from build123d import *

# Parameters (mm, degrees)
SKETCH1_R            = 28.4
BOSS_EXTRUDE1_DEPTH  = 26
SKETCH2_OUTSIDE_W    = 75.686
SKETCH2_OUTSIDE_H    = 75.686
SKETCH2_OUTSIDE_R    = 15
CUT_EXTRUDE1_DEPTH   = 20
CUT_EXTRUDE2_DEPTH   = 48.844748928
CHAMFER1_SIZE        = 0.5
M5_CLEARANCE_HOLE1_D = 5.5
CIRPATTERN1_COUNT    = 6
SKETCH9_R            = 4
CUT_EXTRUDE3_DEPTH   = 48.844748928


with BuildPart() as part:
    # Sketch1 → Boss-Extrude1 (new body)
    with BuildSketch(Plane.XY):
        with Locations(Location((0, 0, 0), (0, 0, 180))):
            Circle(SKETCH1_R)
    extrude(amount=BOSS_EXTRUDE1_DEPTH)

    # Sketch2 outside → Cut-Extrude1 (cut)
    with BuildSketch(Plane(origin=(0, 0, 0), x_dir=(-1, 0, 0), z_dir=(0, 0, -1))):
        Rectangle(SKETCH2_OUTSIDE_W, SKETCH2_OUTSIDE_H)
        Circle(SKETCH2_OUTSIDE_R, mode=Mode.SUBTRACT)
    extrude(amount=-CUT_EXTRUDE1_DEPTH, mode=Mode.SUBTRACT)

    # Sketch3 → Cut-Extrude2 (cut, through all)
    with BuildSketch(Plane(origin=(0, 0, 0), x_dir=(-1, 0, 0), z_dir=(0, 0, -1))):
        with BuildLine():
            Line((2.5, -6.538348415), (2.5, -9.3))
            Line((2.5, -9.3), (-2.5, -9.3))
            Line((-2.5, -9.3), (-2.5, -6.538348415))
            ThreePointArc((-2.5, -6.538348415), (0, 7), (2.5, -6.538348415))
        make_face()
    extrude(amount=-CUT_EXTRUDE2_DEPTH, mode=Mode.SUBTRACT)

    # Chamfer1
    chamfer1_edges = [part.edges().sort_by_distance(p)[0] for p in [
        (28.4, 0, 26),
        (28.4, 0, 20),
    ]]
    chamfer(chamfer1_edges, length=CHAMFER1_SIZE)

    # M5 Clearance Hole1 (through all)
    with Locations(Plane.XY.offset(26)):
        with Locations((23.75, 0)):
            m5_clearance_hole1 = Hole(M5_CLEARANCE_HOLE1_D / 2)

    # CirPattern1: M5 Clearance Hole1 ×6 about axis
    cirpattern1_axis = Axis((0, 0, 0), (0, 0, 1))
    for i in range(1, CIRPATTERN1_COUNT):
        add(m5_clearance_hole1.rotate(cirpattern1_axis, i * 360 / CIRPATTERN1_COUNT), mode=Mode.SUBTRACT)

    # Sketch9 → Cut-Extrude3 (cut, through all)
    with BuildSketch(Plane(origin=(0, 0, 0), x_dir=(0, 0, -1), z_dir=(1, 0, 0))):
        with Locations((-10.2, 0)):
            Circle(SKETCH9_R)
    extrude(amount=-CUT_EXTRUDE3_DEPTH, mode=Mode.SUBTRACT)


solid = part.part
CAD build for the part. Positions are in the model's coordinates, mm. A direction names the side the tool comes from. Round coordinates to 2 decimals unless told otherwise and drop trailing zeros. Loops run counter-clockwise (first coordinate to the right, second up) from the corner with the lowest first, then second, coordinate; pieces in that order, holes last. Notation, with made-up numbers: (69, 44) - (116, 44) arc R9 ccw to (116, 49) - close; hole circle Ø8 at (-17, 41). An arc over 180 degrees is marked (long way). Put each result on its own line as item: value.
1. Two-plate mould, pull along X, no slides. Class faces 4 (the flat face through (-3.1, 6.5, 0)), 5 (the cylindrical face through (13.144, -18.128, 22.958)), 6 (the cylindrical face through (3.697, -28.158, 22.965)): released by +X, released by -X, zero draft, split by the parting line, or undercut.
Geometry check:
face 4: zero draft
face 5: undercut
face 6: split by the parting line
2. Slice it at A-A on x = 0. List the corners of the cut face in (y, z), and give its area (4 significant figures).
Geometry check:
outline: (-28.4, 20.5) - (-27.9, 20) - (-15, 20) - (-15, 0) - (-9.3, 0) - (-9.3, 26) - (-27.9, 26) - (-28.4, 25.5) - close; (7, 0) - (15, 0) - (15, 20) - (27.9, 20) - (28.4, 20.5) - (28.4, 25.5) - (27.9, 26) - (7, 26) - close
area: 516.5 mm²
3. Slice it at B-B on y = 0. List the corners of the cut face in (x, z), and give its area (3 significant figures).
Geometry check:
outline: (-28.4, 20.5) - (-27.9, 20) - (-26.5, 20) - (-26.5, 26) - (-27.9, 26) - (-28.4, 25.5) - close; (-21, 20) - (-15, 20) - (-15, 14.2) - (-7, 14.2) - (-7, 26) - (-21, 26) - close; (-15, 0) - (-7, 0) - (-7, 6.2) - (-15, 6.2) - close; (7, 0) - (15, 0) - (15, 20) - (21, 20) - (21, 26) - (7, 26) - close; (26.5, 20) - (27.9, 20) - (28.4, 20.5) - (28.4, 25.5) - (27.9, 26) - (26.5, 26) - close
area: 446 mm²
4. Slice it at C-C on z = 3. List the corners of the cut face in (x, y).
Geometry check:
outline: circle Ø30 at (0, 0); hole (-2.5, -9.3) - (2.5, -9.3) - (2.5, -6.54) arc R7 ccw (long way) to (-2.5, -6.54) - close
5. Wall check: line 1 (Z direction, x = -8.5, y = 0); line 2 (Z direction, x = 19, y = 12.5); line 3 (Y direction, x = 0, z = 6.5). Give the ranges that are in metal, low to high.
Geometry check:
line 1: 0 to 6.2, 14.2 to 26
line 2: 20 to 26
line 3: -15 to -9.3, 7 to 15
6. 3-axis set-ups, long thin cutter, end or side, ignore diameter. For faces 1 (the flat face through (-12, -12, 20)), 2 (the flat face through (0, -9.3, 13)), 3 (the cylindrical face through (-10.307, -1.532, 6.505)): which of +Z, -Z, +X, -X, +Y, -Y reach the whole face in a straight line?
Geometry check:
face 1: -Z
face 2: +Z, -Z
face 3: -X
7. Slice it at D-D on z = 23.25. List the corners of the cut face in (x, y) (3 decimals).
Geometry check:
outline: circle Ø56.8 at (0, 0); hole circle Ø5.5 at (-23.75, 0); hole circle Ø5.5 at (-11.875, -20.568); hole circle Ø5.5 at (-11.875, 20.568); hole (-2.5, -9.3) - (2.5, -9.3) - (2.5, -6.538) arc R7 ccw (long way) to (-2.5, -6.538) - close; hole circle Ø5.5 at (11.875, -20.568); hole circle Ø5.5 at (11.875, 20.568); hole circle Ø5.5 at (23.75, 0)
8. Pin check, flat tips, straight feed: P1, Ø1, axis at x = -4, z = 13.5, coming from the -Y side; P2, Ø1, axis at x = 0, z = 6, coming from the -Y side; P3, Ø3, axis at y = -8, z = 11, coming from the +X side. Stop position of each tip, or through.
Geometry check:
P1: y = -14.59
P2: y = -15
P3: x = 13.52
